```python
from build123d import *

# Parameters (mm, degrees)
SKETCH1_R           = 11.05
SKETCH1_R_2         = 1.5
SKETCH1_R_3         = 2
SKETCH1_R_4         = 2.75
BOSS_EXTRUDE1_DEPTH = 10


with BuildPart() as part:
    # Sketch1 → Boss-Extrude1 (new body)
    with BuildSketch(Plane.XY):
        Polygon((0, -60), (0, 60), (-100, 60), (-120, 40), (-120, -40), (-100, -60), align=None)
        with Locations((-98.5, 0)):
            Circle(SKETCH1_R, mode=Mode.SUBTRACT)
        with Locations((-83, 15.5)):
            Circle(SKETCH1_R_2, mode=Mode.SUBTRACT)
        with Locations((-114, 15.5)):
            Circle(SKETCH1_R_2, mode=Mode.SUBTRACT)
        with Locations((-114, -15.5)):
            Circle(SKETCH1_R_2, mode=Mode.SUBTRACT)
        with Locations((-83, -15.5)):
            Circle(SKETCH1_R_2, mode=Mode.SUBTRACT)
        with Locations((-60.75, 37.5)):
            Circle(SKETCH1_R_3, mode=Mode.SUBTRACT)
        with Locations((-29.25, 37.5)):
            Circle(SKETCH1_R_3, mode=Mode.SUBTRACT)
        with Locations((-60.75, 11.5)):
            Circle(SKETCH1_R_3, mode=Mode.SUBTRACT)
        with Locations((-29.25, 11.5)):
            Circle(SKETCH1_R_3, mode=Mode.SUBTRACT)
        with Locations((-60.75, -11.5)):
            Circle(SKETCH1_R_3, mode=Mode.SUBTRACT)
        with Locations((-29.25, -11.5)):
            Circle(SKETCH1_R_3, mode=Mode.SUBTRACT)
        with Locations((-29.25, -37.5)):
            Circle(SKETCH1_R_3, mode=Mode.SUBTRACT)
        with Locations((-60.75, -37.5)):
            Circle(SKETCH1_R_3, mode=Mode.SUBTRACT)
        with Locations((-15, 47)):
            Circle(SKETCH1_R_4, mode=Mode.SUBTRACT)
        with Locations((-15, 15)):
            Circle(SKETCH1_R_4, mode=Mode.SUBTRACT)
        with Locations((-15, -15)):
            Circle(SKETCH1_R_4, mode=Mode.SUBTRACT)
        with Locations((-15, -47)):
            Circle(SKETCH1_R_4, mode=Mode.SUBTRACT)
    extrude(amount=BOSS_EXTRUDE1_DEPTH)


solid = part.part
```
Build history of the part. All positions in model axes, mm. Round coordinates to 2 decimals unless told otherwise and drop trailing zeros. Loops run counter-clockwise (first coordinate to the right, second up) from the corner with the lowest first, then second, coordinate; pieces in that order, holes last.
Item 1: Saw through at B-B (y = -7). List the corners of the cut face in (x, z), then the cut area to 3 significant figures.
Item 2: Drill centre lines: line 1 along Y through (x, z) = (-15, 3.5); line 2 along Y through (x, z) = (-60.75, 4.25); line 3 along Y through (x, z) = (-98.5, 6.75). Where is each one in solid material? Low to high.
Item 3: Saw through at C-C (x = -98.5). List the corners of the cut face in (y, z).
Item 4: Pin check, flat tip, straight feed: P1, Ø2.5, axis at x = -114, y = 15.5, coming from the +Z side. Stop position of the tip, or through.
Item 5: Saw through at A-A (x = -15). List the corners of the cut face in (y, z).
Item 6: Two-plate mould, pull along Y, no slides. Class faces 1 (the face through (0, -1, 5)), 2 (the face through (-110, 50, 5)), 3 (the face through (-61.184, -39.452, 4.93)), 4 (the face through (-110, -50, 5)): released by +Y, released by -Y, zero draft, split by the parting line, or undercut.
Item 7: Saw through at D-D (z = 5.5). State how many separate pieces and enclosed holes the cut face has, then the cut area to 3 significant figures.
Worked answers:
1. outline: (-120, 0) - (-107.05, 0) - (-107.05, 10) - (-120, 10) - close; (-89.95, 0) - (0, 0) - (0, 10) - (-89.95, 10) - close
1. area: 1,030 mm2
2. line 1: y = -60 to -49.75, -44.25 to -17.75, -12.25 to 12.25, 17.75 to 44.25, 49.75 to 60
2. line 2: y = -60 to -39.5, -35.5 to -13.5, -9.5 to 9.5, 13.5 to 35.5, 39.5 to 60
2. line 3: y = -60 to -11.05, 11.05 to 60
3. outline: (-60, 0) - (-11.05, 0) - (-11.05, 10) - (-60, 10) - close; (11.05, 0) - (60, 0) - (60, 10) - (11.05, 10) - close
4. P1: passes through
5. outline: (-60, 0) - (-49.75, 0) - (-49.75, 10) - (-60, 10) - close; (-44.25, 0) - (-17.75, 0) - (-17.75, 10) - (-44.25, 10) - close; (-12.25, 0) - (12.25, 0) - (12.25, 10) - (-12.25, 10) - close; (17.75, 0) - (44.25, 0) - (44.25, 10) - (17.75, 10) - close; (49.75, 0) - (60, 0) - (60, 10) - (49.75, 10) - close
6. face 1: zero draft
6. face 2: released by +Y
6. face 3: undercut
6. face 4: released by -Y
7. separate pieces: 1
7. enclosed holes: 17
7. area: 13,400 mm2
